Source: three-view drawing plus pictorial views. Frame: mm from the lowest corner of the part. Give positions to 0.01 mm unless a question says otherwise; leave off trailing zeros. Order: outer loops, then holes, each group sorted by start corner. A loop starts at its lowest first (then second) coordinate and runs counter-clockwise, first axis right, second up. Notation, with made-up numbers: (-10.5, -2.75) -> (36.5, -2.75) arc R25 ccw to (36.5, 20.25) -> close; hole circle Ø8 at (56.25, -22). An arc over 180 degrees is marked (long way). Write item = value, one per line.
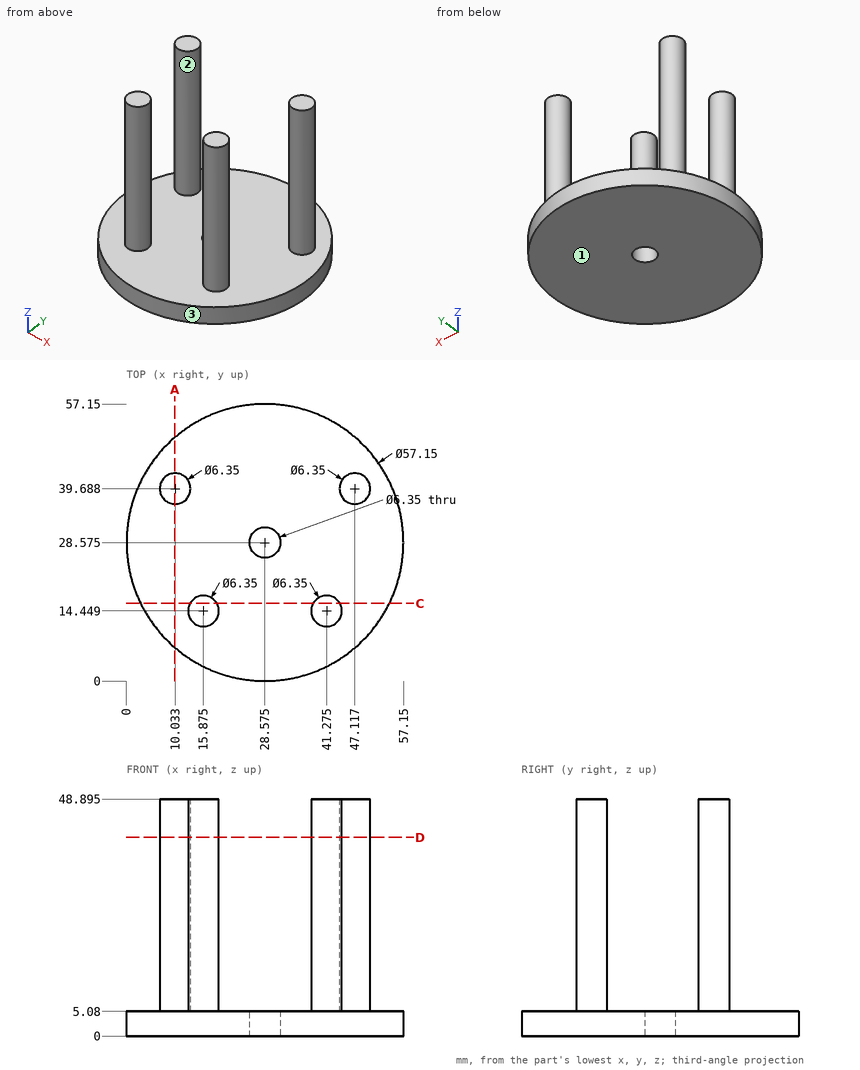
1) Section query C-C (y = 16). Output: boundary loops of the cut face in (x, z) (1 decimal).
Check sheet entries:
outline = (2.9, 0) -> (54.2, 0) -> (54.2, 5.1) -> (44, 5.1) -> (44, 48.9) -> (38.5, 48.9) -> (38.5, 5.1) -> (18.6, 5.1) -> (18.6, 48.9) -> (13.1, 48.9) -> (13.1, 5.1) -> (2.9, 5.1) -> close
2) Mould query, pull axis X, two halves, no side actions, for the marked faces 1, 2 and 3. Classes: +X half, -X half, draft (parallel to the pull), parting line (faces both ways), or undercut.
Check sheet entries:
face_1 = draft
face_2 = undercut
face_3 = parting line
3) First-contact query: P1, Ø12, axis at y = 8.5, z = 40, coming from the -X side; P2, Ø8, axis at y = 45, z = 38, coming from the -X side; P3, Ø4, axis at x = 14, z = 16.5, coming from the +Y side. Flat tips, straight axial feed; report the tip coordinate or a pass-through.
Check sheet entries:
P1 = 12.7
P2 = 7.14
P3 = 42.18
4) Section query A-A (x = 10). Output: boundary loops of the cut face in (y, z) (1 decimal).
Check sheet entries:
outline = (6.9, 0) -> (50.3, 0) -> (50.3, 5.1) -> (42.9, 5.1) -> (42.9, 48.9) -> (36.5, 48.9) -> (36.5, 5.1) -> (6.9, 5.1) -> close
5) Section query D-D (z = 41). Count the separate pieces of the cut face and the enclosed holes in it, plus the area to 3 significant figures.
Check sheet entries:
separate_pieces = 4
enclosed_holes = 0
area = 127 mm²
6) Line query: line 1 (Z direction, x = 38, y = 22); line 2 (X direction, y = 13.5, z = 9) (1 decimal); line 3 (X direction, y = 39.5, z = 26). Output: solid intervals per line, ascending. Write a range as from..to.
Check sheet entries:
line_1 = 0..5.08
line_2 = 12.8..18.9, 38.2..44.3
line_3 = 6.86..13.2, 43.95..50.29
